Could you check a few things on this model? Use its own coordinates, in mm. A direction names the side the tool comes from. Round coordinates to 2 decimals unless told otherwise and drop trailing zeros. Write each loop counter-clockwise with the first axis right and the second up, starting at its lowest first coordinate (ties: lowest second). Pieces come first, ordered by that corner, then holes. Notation, with made-up numbers: (-33.5, 17) -> (-18.5, 17) arc R18 cw to (-18.5, 34) -> close; hole circle Ø9 at (48.5, 35). An arc over 180 degrees is marked (long way). Return JSON: item names as keys, results as strings.
from build123d import *

# Parameters (mm, degrees)
SKETCH1_W            = 70
SKETCH1_H            = 95
BASE_DEPTH           = 28
SKETCH1_7_W          = 10
SKETCH1_7_H          = 10
SKETCH1_7_R          = 1.5
MOUNTING_HOLES_DEPTH = 5
SKETCH1_6_W          = 60
SKETCH1_6_H          = 85
SKETCH1_6_R          = 2.85
SKETCH1_6_R_2        = 1.85
CAVITY_DEPTH         = 25
STANDOFF_START       = 25
SKETCH1_9_R          = 2.85
SKETCH1_9_R_2        = 1.85
STANDOFF_DEPTH       = 3
PG9_DEPTH            = 5
SKETCH3_3_R          = 11.414954575
SKETCH3_3_R_2        = 8
CUT_EXTRUDE4_DEPTH   = 3
EXTERNAL_FILLET_R    = 1.5


with BuildPart() as part:
    # Sketch1 → Base (new body)
    with BuildSketch(Plane.XY):
        Rectangle(SKETCH1_W, SKETCH1_H)
    extrude(amount=BASE_DEPTH)

    # Sketch1<7> → Mounting Holes (add)
    # profile 1 of 4: a face of its own
    with BuildSketch(Plane.XY):
        with Locations((40, 39.5)):
            Rectangle(SKETCH1_7_W, SKETCH1_7_H)
        with Locations((40, 39.5)):
            Circle(SKETCH1_7_R, mode=Mode.SUBTRACT)
    # profile 2 of 4: a face of its own
    with BuildSketch(Plane.XY):
        with Locations((40, -39.5)):
            Rectangle(SKETCH1_7_W, SKETCH1_7_H)
        with Locations((40, -39.5)):
            Circle(SKETCH1_7_R, mode=Mode.SUBTRACT)
    # profile 3 of 4: a face of its own
    with BuildSketch(Plane.XY):
        with Locations((-40, -39.5)):
            Rectangle(SKETCH1_7_W, SKETCH1_7_H)
        with Locations((-40, -39.5)):
            Circle(SKETCH1_7_R, mode=Mode.SUBTRACT)
    # profile 4 of 4: a face of its own
    with BuildSketch(Plane.XY):
        with Locations((-40, 39.5)):
            Rectangle(SKETCH1_7_W, SKETCH1_7_H)
        with Locations((-40, 39.5)):
            Circle(SKETCH1_7_R, mode=Mode.SUBTRACT)
    extrude(amount=MOUNTING_HOLES_DEPTH)

    # Sketch1<6> → Cavity (cut)
    # profile 1 of 5: a face of its own
    with BuildSketch(Plane.XY):
        Rectangle(SKETCH1_6_W, SKETCH1_6_H)
        with Locations((0.70771822, -25.5)):
            Circle(SKETCH1_6_R, mode=Mode.SUBTRACT)
        with Locations((0.70771822, 27.586)):
            Circle(SKETCH1_6_R, mode=Mode.SUBTRACT)
    # profile 2 of 5: a face of its own
    with BuildSketch(Plane.XY):
        with Locations((0.70771822, 27.586)):
            Circle(SKETCH1_6_R)
        with Locations((0.70771822, 27.586)):
            Circle(SKETCH1_6_R_2, mode=Mode.SUBTRACT)
    # profile 3 of 5: a face of its own
    with BuildSketch(Plane.XY):
        with Locations((0.70771822, 27.586)):
            Circle(SKETCH1_6_R_2)
    # profile 4 of 5: a face of its own
    with BuildSketch(Plane.XY):
        with Locations((0.70771822, -25.5)):
            Circle(SKETCH1_6_R)
        with Locations((0.70771822, -25.5)):
            Circle(SKETCH1_6_R_2, mode=Mode.SUBTRACT)
    # profile 5 of 5: a face of its own
    with BuildSketch(Plane.XY):
        with Locations((0.70771822, -25.5)):
            Circle(SKETCH1_6_R_2)
    extrude(amount=CAVITY_DEPTH, mode=Mode.SUBTRACT)

    # Sketch1<9> → Standoff (add)
    # profile 1 of 2: a face of its own
    with BuildSketch(Plane.XY.offset(STANDOFF_START)):
        with Locations((0.70771822, 27.586)):
            Circle(SKETCH1_9_R)
        with Locations((0.70771822, 27.586)):
            Circle(SKETCH1_9_R_2, mode=Mode.SUBTRACT)
    # profile 2 of 2: a face of its own
    with BuildSketch(Plane.XY.offset(STANDOFF_START)):
        with Locations((0.70771822, -25.5)):
            Circle(SKETCH1_9_R)
        with Locations((0.70771822, -25.5)):
            Circle(SKETCH1_9_R_2, mode=Mode.SUBTRACT)
    extrude(amount=-STANDOFF_DEPTH)

    # Sketch3 → PG9 (cut)
    with BuildSketch(Plane(origin=(7.707718219, 47.5, 0), x_dir=(0, 0, 1), z_dir=(0, -1, 0))):
        with BuildLine():
            ThreePointArc((4.5, 7.707718219), (12.5, -0.292281781), (20.5, 7.707718219))
            Line((20.5, 7.707718219), (4.5, 7.707718219))
        make_face()
        with BuildLine():
            Line((4.5, 7.707718219), (20.5, 7.707718219))
            ThreePointArc((20.5, 7.707718219), (12.5, 15.707718219), (4.5, 7.707718219))
        make_face()
    extrude(amount=PG9_DEPTH, mode=Mode.SUBTRACT)

    # Sketch3<3> → Cut-Extrude4 (cut)
    with BuildSketch(Plane(origin=(7.707718219, 47.5, 0), x_dir=(0, 0, 1), z_dir=(0, -1, 0))):
        with Locations(Location((12.5, 7.707718219, 0), (0, 0, 90))):
            Circle(SKETCH3_3_R)
        with Locations((12.5, 7.707718219)):
            Circle(SKETCH3_3_R_2, mode=Mode.SUBTRACT)
    extrude(amount=CUT_EXTRUDE4_DEPTH, mode=Mode.SUBTRACT)

    # External Fillet
    external_fillet_edges = [part.edges().sort_by_distance(p)[0] for p in [
        (45, 34.5, 2.5),
        (45, 44.5, 2.5),
        (35, 39.5, 5),
        (35, 44.5, 2.5),
        (35, 34.5, 2.5),
        (45, -34.5, 2.5),
        (35, -39.5, 5),
        (35, -34.5, 2.5),
        (35, -44.5, 2.5),
        (45, -44.5, 2.5),
        (-45, -34.5, 2.5),
        (-45, -44.5, 2.5),
        (-35, -44.5, 2.5),
        (-35, -34.5, 2.5),
        (-35, -39.5, 5),
        (-35, 34.5, 2.5),
        (-35, 44.5, 2.5),
        (-45, 44.5, 2.5),
        (-45, 34.5, 2.5),
        (-35, 39.5, 5),
        (-35, -47.5, 14),
        (-35, 47.5, 14),
        (35, 47.5, 14),
        (35, -47.5, 14),
    ]]
    fillet(external_fillet_edges, radius=EXTERNAL_FILLET_R - 0.0001)  # a hair under: the kernel refuses the full size


solid = part.part
1) Thinking about a two-plate mould opening in X: for faces 1 (the face through (45, -40, 2)), 2 (the face through (0, 1, 28)), 3 (the face through (-2.4, 44.5, 4.7)), which applies, pulls with the +X half, pulls with the -X half, needs draft (parallel to the pull), parting line crosses it, or undercut?
Return value:
{"face 1": "pulls with the +X half", "face 2": "needs draft", "face 3": "undercut"}
2) If I drill on probe 1 along Y at (x, z) = (-40, 2.65); probe 2 along Y at (x, z) = (-14, 21.5); probe 3 along X at (y, z) = (16.5, 22), over which ranges is the centre line in solid material (lowest first)? Write a range as [from, to].
Return value:
{"probe 1": "[-44.5, -41], [-38, -34.5], [34.5, 38], [41, 44.5]", "probe 2": "[-47.5, -42.5], [42.5, 47.5]", "probe 3": "[-35, -30], [30, 35]"}
3) Will these pins go through, and if not, where does the flat tip stop? pin 1 Ø12.5 at (y, z) = (11.5, 13.5) entering from -X; pin 2 Ø12 at (y, z) = (12, 18.5) entering from +X; pin 3 Ø3 at (y, z) = (-35.5, 7.5) entering from -X; pin 4 Ø2.5 at (x, y) = (-40, -39.5) entering from -Z.
Return value:
{"pin 1": "x = -35", "pin 2": "x = 35", "pin 3": "x = -35.09", "pin 4": "through"}
4) For faces 4 (the face through (-40, 44.5, 2)), 5 (the face through (0.47, 29.42, 23.52)), 6 (the face through (40, -44.5, 2)), which set-ups out of +Z, -Z, +X, -X, +Y, -Y let a thin tool reach every point of the face, with its end or its side?
Return value:
{"face 4": "+Z, -Z, -X, +Y", "face 5": "-Z", "face 6": "+Z, -Z, +X, -Y"}
5) I want a section at C-C, the plane y = 10.5. Please give me the cut outline in (x, z), and give its area (3 significant figures).
Return value:
{"outline": "(-35, 0) -> (-30, 0) -> (-30, 25) -> (30, 25) -> (30, 0) -> (35, 0) -> (35, 28) -> (-35, 28) -> close", "area": "460 mm²"}
6) I want a section at B-B, the plane x = -4. Please give me the cut outline in (y, z), and give its area (3 significant figures).
Return value:
{"outline": "(-47.5, 0) -> (-42.5, 0) -> (-42.5, 25) -> (42.5, 25) -> (42.5, 19.43) -> (44.5, 19.43) -> (44.5, 23.19) -> (47.5, 23.19) -> (47.5, 28) -> (-47.5, 28) -> close; (42.5, 0) -> (47.5, 0) -> (47.5, 1.81) -> (44.5, 1.81) -> (44.5, 5.57) -> (42.5, 5.57) -> close", "area": "443 mm²"}
7) I want a section at D-D, the plane z = 12.5. Please give me the cut outline in (x, y).
Return value:
{"outline": "(-35, -46) arc R1.5 ccw to (-33.5, -47.5) -> (33.5, -47.5) arc R1.5 ccw to (35, -46) -> (35, 46) arc R1.5 ccw to (33.5, 47.5) -> (11.41, 47.5) -> (11.41, 44.5) -> (8, 44.5) -> (8, 42.5) -> (30, 42.5) -> (30, -42.5) -> (-30, -42.5) -> (-30, 42.5) -> (-8, 42.5) -> (-8, 44.5) -> (-11.41, 44.5) -> (-11.41, 47.5) -> (-33.5, 47.5) arc R1.5 ccw to (-35, 46) -> close"}
8) I want a section at A-A, the plane y = -39.5. Please give me the cut outline in (x, z), and give its area (3 significant figures).
Return value:
{"outline": "(-45, 0) -> (-41.5, 0) -> (-41.5, 5) -> (-45, 5) -> close; (-38.5, 0) -> (-30, 0) -> (-30, 25) -> (30, 25) -> (30, 0) -> (38.5, 0) -> (38.5, 5) -> (36.5, 5) arc R1.5 cw to (35, 6.5) -> (35, 28) -> (-35, 28) -> (-35, 6.5) arc R1.5 cw to (-36.5, 5) -> (-38.5, 5) -> close; (41.5, 0) -> (45, 0) -> (45, 5) -> (41.5, 5) -> close", "area": "531 mm²"}
